Read the model definition and answer for the solid it produces. Units are mm, in the model's axes. A direction names the side the tool comes from. Coordinates: 2 decimals unless noted, no trailing zeros. Write each loop counter-clockwise with the first axis right and the second up, starting at its lowest first coordinate (ties: lowest second). Pieces come first, ordered by that corner, then holes.
(1) Find the intervals of material crossed by probe 1 along X at (y, z) = (0.8, -80.5); probe 2 along Z at (x, y) = (-33.5, 0.65); probe 3 along X at (y, z) = (1, -5), in increasing order.
(2) The mould has two halves that part along Z. Classify faces 5 (the flat face through (-20, -22, -43)), 6 (the flat face through (-19, 7, -28.5)), 7 (the flat face through (-20, -11, -82)): +Z half, -Z half, draft (parallel to the pull), parting line (faces both ways), or undercut.
(3) Section A-A on x = -23.5 is taken. Write down the section's boundary in (y, z), then the cut area to 3 significant figures.
(4) Section C-C on y = -3 is taken. Write down the section's boundary in (x, z).
(5) Given pin 1 (1.5 mm diameter, centred on x = -25.5, y = 3.5, fed in from +Z); pin 2 (8 mm diameter, centred on y = -14.5, z = -46, fed in from +X); pin 3 (8 mm diameter, centred on y = 7, z = -54.5, fed in from +X); pin 4 (5.5 mm diameter, centred on y = 4, z = -14.5, fed in from -X), each flat-ended and moving along its own axis, determine where each tip first touches the part or whether it passes through.
(6) Section B-B on z = -13 is taken. Write down the section's boundary in (x, y), then the cut area to 3 significant figures.
(7) Section D-D on z = -34.5 is taken. Write down the section's boundary in (x, y), then the cut area to 3 significant figures.
(8) Which of the six approach directions +Z, -Z, +X, -X, +Y, -Y give full straight-line access (tool end or side, diameter ignored) to faces 1 (the flat face through (-9.5, -11, -44)), 2 (the flat face through (-19, -11, -4.5)), 3 (the flat face through (-29.5, -11, -43)), 4 (the flat face through (-32.25, 7, -52))?
Autodesk Inventor part; units mm, degrees
ref_plane "YZ Plane" through (0, 0, 0) normal (1, 0, 0) x (0, 1, 0)
ref_plane "XZ Plane" through (0, 0, 0) normal (0, 1, 0) x (-1, 0, 0)
ref_plane "XY Plane" through (0, 0, 0) normal (0, 0, 1) x (1, 0, 0)
sketch "Sketch1" plane through (0, 0, 0) normal (0, 1, 0) x (-1, 0, 0)
  line L0 (5, 0) -> (33.5, 0)
  line L1 (38.5, -5) -> (38.5, -80.5)
  line L2 (33.5, -85.5) -> (5, -85.5)
  line L3 (0, -80.5) -> (0, -5)
  arc A0 (38.5, -5) -> (33.5, 0) centre (33.5, -5) ccw
  arc A1 (33.5, -85.5) -> (38.5, -80.5) centre (33.5, -80.5) ccw
  arc A2 (0, -80.5) -> (5, -85.5) centre (5, -80.5) ccw
  arc A3 (5, 0) -> (0, -5) centre (5, -5) ccw
  point P0 (0, 0)
  point P1 (38.5, -85.5)
  point P2 (38.5, 0)
  point P3 (0, -85.5)
  dimension "d0" = 38.5
  dimension "d1" = 85.5
  dimension "d2" = 5
  dimension "d3" = 5
  dimension "d4" = 5
  dimension "d5" = 5
extrude "Extrusion1" add sketch "Sketch1" along normal blind 1.6
sketch "Sketch2" plane through (0, 1.6, 0) normal (0, 1, 0) x (1, 0, 0)
  arc A0 (-5, 0) -> (0, 5) centre (-5, 5) ccw
  arc A1 (0, 80.5) -> (-5, 85.5) centre (-5, 80.5) ccw
  circle A2 centre (-5, 80.5) radius 1.6
  arc A3 (-33.5, 85.5) -> (-38.5, 80.5) centre (-33.5, 80.5) ccw
  circle A4 centre (-33.5, 80.5) radius 1.6
  arc A5 (-38.5, 5) -> (-33.5, 0) centre (-33.5, 5) ccw
  circle A6 centre (-33.5, 5) radius 1.6
  point P0 (0, 0)
  dimension "d9" = 3.2
  dimension "d10" = 3.2
  dimension "d11" = 3.2
extrude "Extrusion2" cut sketch "Sketch2" against normal blind 35
sketch "Sketch4" plane through (0, 0, 0) normal (0, -1, 0) x (1, 0, 0)
  line L0 (0, 0) -> (-9.5, 0)
  line L1 (-9.5, 0) -> (-9.5, -4.5)
  line L2 (-9.5, -4.5) -> (0, -4.5)
  line L3 (0, -4.5) -> (0, 0)
  line L4 (-9.5, -4.5) -> (-29.5, -4.5)
  line L5 (-29.5, -4.5) -> (-29.5, -82)
  line L6 (-29.5, -82) -> (-9.5, -82)
  line L7 (-9.5, -82) -> (-9.5, -4.5)
  dimension "d14" = 9.5
  dimension "d15" = 4.5
  dimension "d16" = 20
  dimension "d17" = 77.5
extrude "Extrusion3" add sketch "Sketch4" along normal blind 22 contours L7 L6 L5 L4
sketch "Sketch5" plane through (0, 1.6, 0) normal (0, 1, 0) x (1, 0, 0)
  line L0 (0, 0) -> (-10.5, 0)
  line L1 (-10.5, 0) -> (-10.5, 9.5)
  line L2 (-10.5, 9.5) -> (0, 9.5)
  line L3 (0, 9.5) -> (0, 0)
  line L4 (-10.5, 9.5) -> (-38, 9.5)
  line L5 (-38, 9.5) -> (-38, 27)
  line L6 (-38, 27) -> (-10.5, 27)
  line L7 (-10.5, 27) -> (-10.5, 9.5)
  dimension "d20" = 10.5
  dimension "d21" = 9.5
  dimension "d22" = 27.5
  dimension "d23" = 17.5
extrude "Extrusion4" add sketch "Sketch5" along normal blind 5 contours L4 L5 L6 L7
sketch "Sketch6" plane through (0, 1.6, 0) normal (0, 1, 0) x (1, 0, 0)
  line L0 (0, 0) -> (-6.75, 0)
  line L1 (-6.75, 0) -> (-6.75, 28.5)
  line L2 (-6.75, 28.5) -> (0, 28.5)
  line L3 (0, 28.5) -> (0, 0)
  line L4 (-6.75, 28.5) -> (-32.25, 28.5)
  line L5 (-32.25, 28.5) -> (-32.25, 77)
  line L6 (-32.25, 77) -> (-6.75, 77)
  line L7 (-6.75, 77) -> (-6.75, 28.5)
  dimension "d26" = 6.75
  dimension "d27" = 28.5
  dimension "d28" = 25.5
  dimension "d29" = 48.5
extrude "Extrusion5" add sketch "Sketch6" along normal blind 10 contours L4 L5 L6 L7
properties part number "PCB"
Response:
1. probe 1: x = -38.5 to -35.1, -31.9 to -6.6, -3.4 to 0
1. probe 2: z = -85.5 to -82.1, -78.9 to -6.6, -3.4 to 0
1. probe 3: x = -38.5 to -35.1, -31.9 to 0
2. face 5: draft
2. face 6: undercut
2. face 7: -Z half
3. outline: (-22, -82) - (0, -82) - (0, -85.5) - (1.6, -85.5) - (1.6, -77) - (11.6, -77) - (11.6, -28.5) - (1.6, -28.5) - (1.6, -27) - (6.6, -27) - (6.6, -9.5) - (1.6, -9.5) - (1.6, 0) - (0, 0) - (0, -4.5) - (-22, -4.5) - close
3. area: 2,410 mm2
4. outline: (-29.5, -82) - (-9.5, -82) - (-9.5, -4.5) - (-29.5, -4.5) - close
5. pin 1: stops at z = -9.5
5. pin 2: stops at x = -9.5
5. pin 3: stops at x = -6.75
5. pin 4: stops at x = -38.5
6. outline: (-38.5, 0) - (-29.5, 0) - (-29.5, -22) - (-9.5, -22) - (-9.5, 0) - (0, 0) - (0, 1.6) - (-10.5, 1.6) - (-10.5, 6.6) - (-38, 6.6) - (-38, 1.6) - (-38.5, 1.6) - close
6. area: 639 mm2
7. outline: (-38.5, 0) - (-29.5, 0) - (-29.5, -22) - (-9.5, -22) - (-9.5, 0) - (0, 0) - (0, 1.6) - (-6.75, 1.6) - (-6.75, 11.6) - (-32.25, 11.6) - (-32.25, 1.6) - (-38.5, 1.6) - close
7. area: 757 mm2
8. face 1: +Z, -Z, +X, -Y
8. face 2: +Z, +X, -X, -Y
8. face 3: +Z, -Z, -X, -Y
8. face 4: -Z, -X, +Y
